from build123d import *

# Parameters (mm, degrees)
SKETCH1_W            = 127
SKETCH1_H            = 101.6
BOSS_EXTRUDE1_DEPTH  = 6.35
HOLE2_D              = 17.4625
M4_CLEARANCE_HOLE1_D = 5.5


with BuildPart() as part:
    # Sketch1 → Boss-Extrude1 (new, symmetric)
    with BuildSketch(Plane.XY):
        Rectangle(SKETCH1_W, SKETCH1_H)
    extrude(amount=BOSS_EXTRUDE1_DEPTH, both=True)

    # Hole2 (through all)
    with Locations(Plane.XY.offset(6.35)):
        with Locations((0, -6.35)):
            Hole(HOLE2_D / 2)

    # M4 Clearance Hole1 (through all)
    with Locations(Plane.XY.offset(6.35)):
        with Locations((-10, -40.8), (10, -40.8)):
            Hole(M4_CLEARANCE_HOLE1_D / 2)


solid = part.part
Input: part model. Units: mm. Frame: model coordinates. Give positions to 0.01 mm unless a question says otherwise; leave off trailing zeros. Write each loop counter-clockwise with the first axis right and the second up, starting at its lowest first coordinate (ties: lowest second). Pieces come first, ordered by that corner, then holes.
Q1. Material intervals for probe 1 along Y at (x, z) = (0, 0.25); probe 2 along Y at (x, z) = (-10, 1); probe 3 along Y at (x, z) = (8, -0.75), sorted ascending.
Q2. First-contact query: P1, Ø3.5, axis at x = 10, y = -40.8, coming from the +Z side. Flat tip, straight axial feed; report the tip coordinate or a pass-through.
Q3. Section C-C, the plane z = 1.5. Output: boundary loops of the cut face in (x, y), plus the area to 3 significant figures.
Q4. Section B-B, the plane y = -6.35. Output: boundary loops of the cut face in (x, z), plus the area to 3 significant figures.
Q5. Section A-A, the plane x = 0. Output: boundary loops of the cut face in (y, z).
Q6. Pull-direction query (Y, two-part tool) for faces 1 (the face through (-1, 50.8, 0)), 2 (the face through (-1, -50.8, 0)), 3 (the face through (-9.404, -43.485, -0.089)), 4 (the face through (8.73, -43.24, -0.09)); classes: pulls with the +Y half, pulls with the -Y half, needs draft (parallel to the pull), parting line crosses it, or undercut.
Q7. Section D-D, the plane y = -40.8. Output: boundary loops of the cut face in (x, z).
Filled in:
1. probe 1: y = -50.8 to -15.08, 2.38 to 50.8
1. probe 2: y = -50.8 to -43.55, -38.05 to 50.8
1. probe 3: y = -50.8 to -42.69, -38.91 to -9.85, -2.85 to 50.8
2. P1: passes through
3. outline: (-63.5, -50.8) - (63.5, -50.8) - (63.5, 50.8) - (-63.5, 50.8) - close; hole circle Ø5.5 at (-10, -40.8); hole circle Ø17.46 at (0, -6.35); hole circle Ø5.5 at (10, -40.8)
3. area: 12,600 mm2
4. outline: (-63.5, -6.35) - (-8.73, -6.35) - (-8.73, 6.35) - (-63.5, 6.35) - close; (8.73, -6.35) - (63.5, -6.35) - (63.5, 6.35) - (8.73, 6.35) - close
4. area: 1,390 mm2
5. outline: (-50.8, -6.35) - (-15.08, -6.35) - (-15.08, 6.35) - (-50.8, 6.35) - close; (2.38, -6.35) - (50.8, -6.35) - (50.8, 6.35) - (2.38, 6.35) - close
6. face 1: pulls with the +Y half
6. face 2: pulls with the -Y half
6. face 3: undercut
6. face 4: undercut
7. outline: (-63.5, -6.35) - (-12.75, -6.35) - (-12.75, 6.35) - (-63.5, 6.35) - close; (-7.25, -6.35) - (7.25, -6.35) - (7.25, 6.35) - (-7.25, 6.35) - close; (12.75, -6.35) - (63.5, -6.35) - (63.5, 6.35) - (12.75, 6.35) - close
